Model file for the job. Use its own axes, mm. A direction names the side the tool comes from. Round coordinates to 2 decimals unless told otherwise and drop trailing zeros. Loops run counter-clockwise (first coordinate to the right, second up) from the corner with the lowest first, then second, coordinate; pieces in that order, holes last. Notation, with made-up numbers: M -10.75,-4.5 L 3.25,-4.5 A16 ccw 3.25,17.5 Z; hole C 89.25,-37.5 d11. An arc over 180 degrees is marked long. Use a Markdown table: item, result. Add a question column.
Item 1: Wall check: L1, parallel to Y at x = 0, z = 1.5 (3 decimals); L2, parallel to Y at x = 0, z = 5.2 (3 decimals); L3, parallel to Z at x = -1.5, y = -14. Give the ranges that are in metal, low to high. Write a range as from..to.
Item 2: Saw through at B-B on z = 1.25. Write the cut outline in (x, y) (3 decimals).
Item 3: Pin check, flat tips, straight feed: P1, Ø2.5, axis at x = 1.5, y = 4.5, coming from the +Z side; P2, Ø2.5, axis at x = 0, y = -1.6, coming from the -Z side; P3, Ø6.5, axis at x = -2.5, y = 2.5, coming from the +Z side. Stop position of each tip, or through.
Item 4: Saw through at D-D on y = 5.9. Write the cut outline in (x, z) (3 decimals).
Item 5: Saw through at A-A on y = 13.4. Write the cut outline in (x, z), then the cut area to 3 significant figures.
Item 6: Saw through at C-C on y = -8. Write the cut outline in (x, z), then the cut area to 3 significant figures.
Item 7: Tool access for faces 1 (the flat face through (2, 4, 2.75)), 2 (the flat face through (-4.896, -16.195, 0.247)): list every direction of +Z, -Z, +X, -X, +Y, -Y with a clear straight run to the whole face (end or side of a thin tool).
```python
from build123d import *

# Parameters (mm, degrees)
F0_R     = 2
F0_R_2   = 2.225
F1_DEPTH = 6.1
F2_R     = 3.875
F2_R_2   = 2.225
F3_DEPTH = 3.35
F4_R     = 2
F5_DEPTH = 3
F6_SIZE  = 0.6
F7_SIZE  = 0.5


with BuildPart() as f1:
    # F0 (on Top) → F1 (new body)
    with BuildSketch(Plane.XY):
        Polygon((-7, 14.4), (-7, 0), (-7, -14.4), (-3.1, -18.4), (0, -18.4), (3.1, -18.4), (7, -14.4), (7, 0), (7, 14.4), (3.1, 18.4), (0, 18.4), (-3.1, 18.4), align=None)
        with Locations((0, -1.6)):
            Circle(F0_R, mode=Mode.SUBTRACT)
        with Locations((0, 5.9)):
            Circle(F0_R_2, mode=Mode.SUBTRACT)
        with Locations((0, 13.4)):
            Circle(F0_R, mode=Mode.SUBTRACT)
    extrude(amount=F1_DEPTH)

    # F2 (on face) → F3 (cut)
    with BuildSketch(Plane.XY.offset(6.1)):
        with Locations((0, 5.9)):
            Circle(F2_R)
        with Locations((0, 5.9)):
            Circle(F2_R_2, mode=Mode.SUBTRACT)
    extrude(amount=-F3_DEPTH, mode=Mode.SUBTRACT)

    # F4 (on face) → F5 (join)
    with BuildSketch(Plane.XY.offset(6.1)):
        with Locations((0, -11.4)):
            Circle(F4_R)
    extrude(amount=F5_DEPTH)

    # F6
    f6_edges = [f1.edges().sort_by_distance(p)[0] for p in [
        (-2, -11.4, 9.1),
    ]]
    chamfer(f6_edges, length=F6_SIZE)

    # F7
    f7_edges = [f1.edges().sort_by_distance(p)[0] for p in [
        (-7, 0, 0),
        (-5.05, -16.4, 0),
        (0, -18.4, 0),
        (5.05, -16.4, 0),
        (7, 0, 0),
        (5.05, 16.4, 0),
        (0, 18.4, 0),
        (-5.05, 16.4, 0),
        (5.05, -16.4, 6.1),
        (0, -18.4, 6.1),
        (-5.05, -16.4, 6.1),
        (-7, 0, 6.1),
        (-5.05, 16.4, 6.1),
        (0, 18.4, 6.1),
        (5.05, 16.4, 6.1),
        (7, 0, 6.1),
    ]]
    chamfer(f7_edges, length=F7_SIZE)


solid = f1.part
```
Entries:
| question | item | result |
|---|---|---|
| 1 | L1 | -18.4..-3.6, 0.4..3.675, 8.125..11.4, 15.4..18.4 |
| 1 | L2 | -18.4..-3.6, 0.4..2.025, 9.775..11.4, 15.4..18.4 |
| 1 | L3 | 0..6.1 |
| 2 | outline | M -7,-14.4 L -3.1,-18.4 L 3.1,-18.4 L 7,-14.4 L 7,14.4 L 3.1,18.4 L -3.1,18.4 L -7,14.4 Z; hole C 0,5.9 d4.45; hole C 0,-1.6 d4; hole C 0,13.4 d4 |
| 3 | P1 | z = 2.75 |
| 3 | P2 | through |
| 3 | P3 | z = 6.1 |
| 4 | outline | M -7,0.5 L -6.5,0 L -2.225,0 L -2.225,2.75 L -3.875,2.75 L -3.875,6.1 L -6.5,6.1 L -7,5.6 Z; M 2.225,0 L 6.5,0 L 7,0.5 L 7,5.6 L 6.5,6.1 L 3.875,6.1 L 3.875,2.75 L 2.225,2.75 Z |
| 5 | outline | M -7,0.5 L -6.5,0 L -2,0 L -2,6.1 L -6.5,6.1 L -7,5.6 Z; M 2,0 L 6.5,0 L 7,0.5 L 7,5.6 L 6.5,6.1 L 2,6.1 Z |
| 5 | area | 60.5 mm2 |
| 6 | outline | M -7,0.5 L -6.5,0 L 6.5,0 L 7,0.5 L 7,5.6 L 6.5,6.1 L -6.5,6.1 L -7,5.6 Z |
| 6 | area | 84.9 mm2 |
| 7 | face 1 | +Z |
| 7 | face 2 | -Z, -X, -Y |
